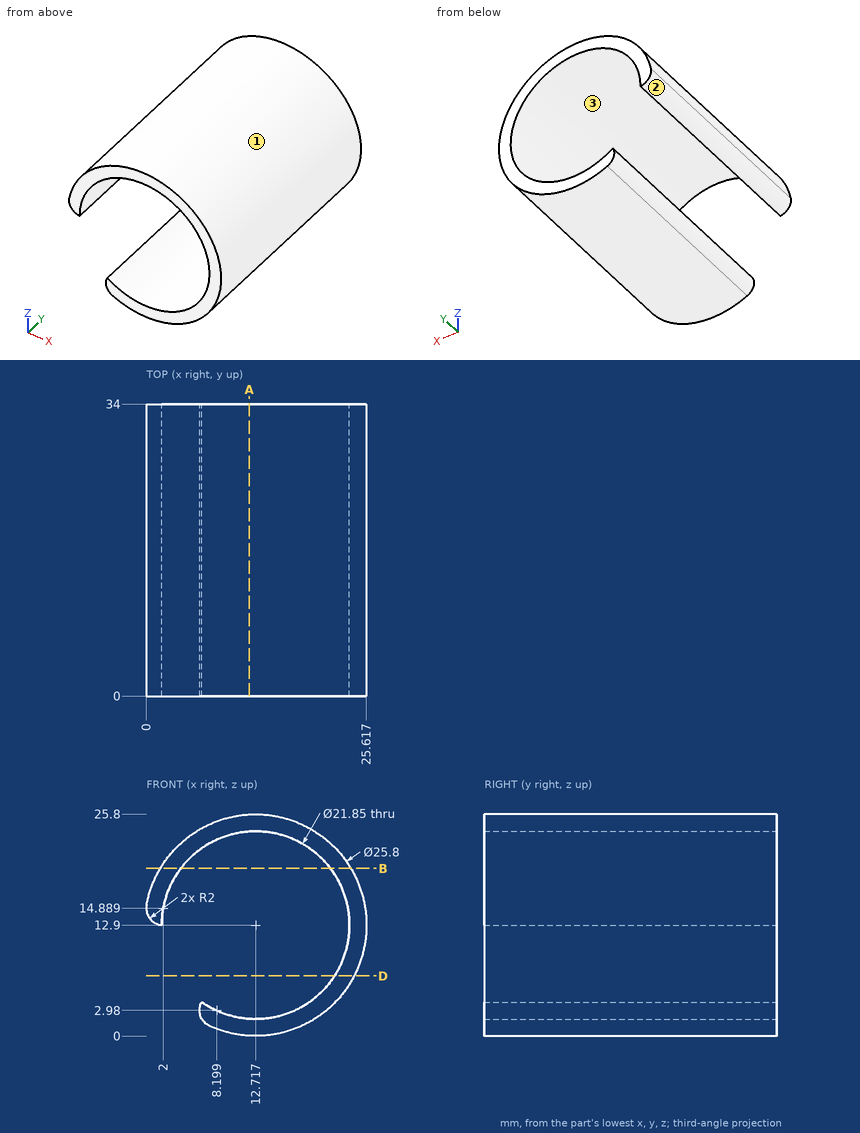
Geometry check sheet. Reference: drawing and pictorial views, mm from the part's lowest x, y, z. Round coordinates to 2 decimals unless told otherwise and drop trailing zeros. Loops run counter-clockwise (first coordinate to the right, second up) from the corner with the lowest first, then second, coordinate; pieces in that order, holes last. Notation, with made-up numbers: (70.5, -9) - (108.5, -9) arc R20 cw to (108.5, 27) - close; hole circle Ø4 at (26, -10). An arc over 180 degrees is marked (long way). Write item = value, one per line. Start each with the question number.
Q1. Section check B-B (z = 19.5). Record the boundary of the cut face in (x, y).
Q2. Section check A-A (x = 12). Record the boundary of the cut face in (y, z).
Q3. Depth check by flat-ended pin: P1, Ø3, axis at y = 12, z = 17, coming from the +X side; P2, Ø4, axis at x = 21.5, y = 23, coming from the +Z side. Enter the tip coordinate at first touch or a pass-through.
Q4. Release check for a two-part mould opening along X. For the marked faces 1, 2 and 3 record: pulls with the +X half, pulls with the -X half, needs draft (parallel to the pull), parting line crosses it, or undercut.
Q5. Section check D-D (z = 7). Record the boundary of the cut face in (x, y).
Q6. Thickness scan on L1, parallel to X at y = 19.5, z = 15 (1 decimal); L2, parallel to X at y = 26, z = 12.5 (1 decimal); L3, parallel to Z at x = 14.5, y = 14.5. Record the ranges inside material, lowest first.
Derived:
q1.outline = (1.63, 0) - (4.01, 0) - (4.01, 34) - (1.63, 34) - close; (21.42, 0) - (23.8, 0) - (23.8, 34) - (21.42, 34) - close
q2.outline = (0, 0.02) - (34, 0.02) - (34, 2) - (0, 2) - close; (0, 23.8) - (34, 23.8) - (34, 25.78) - (0, 25.78) - close
q3.P1 = 25.35
q3.P2 = 23.87
q4.face_1 = parting line crosses it
q4.face_2 = pulls with the -X half
q4.face_3 = undercut
q5.outline = (21.91, 0) - (24.19, 0) - (24.19, 34) - (21.91, 34) - close
q6.L1 = 0 to 2, 23.4 to 25.4
q6.L2 = 23.6 to 25.6
q6.L3 = 0.12 to 2.12, 23.68 to 25.68
